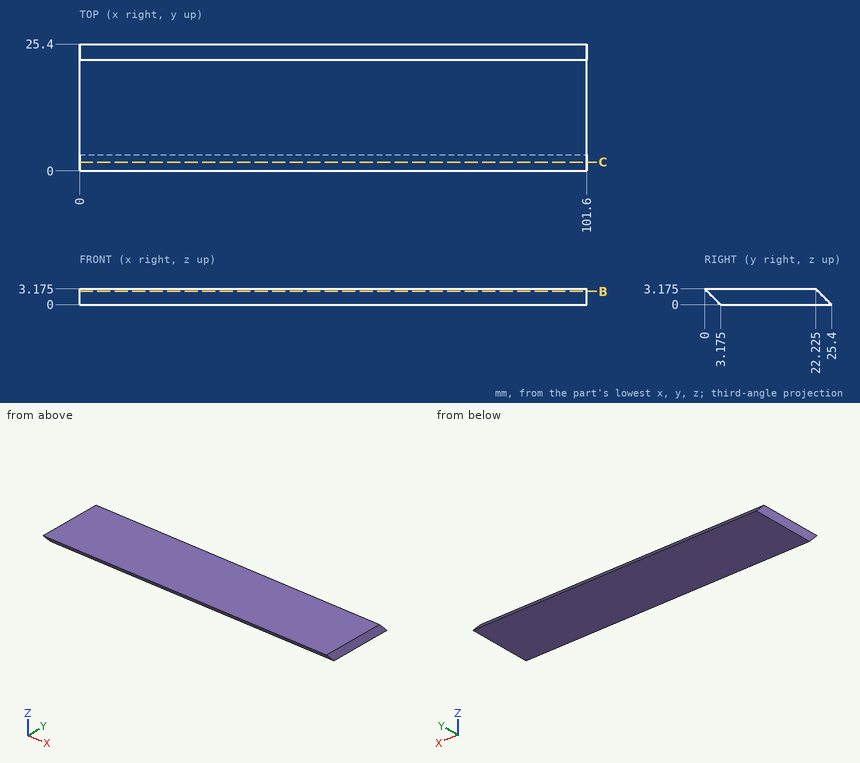
Could you check a few things on this drawing? It's one solid part, dimensions in mm from its lowest x, y, z. Give positions to 0.01 mm unless a question says otherwise; leave off trailing zeros. Order: outer loops, then holes, each group sorted by start corner. A loop starts at its lowest first (then second) coordinate and runs counter-clockwise, first axis right, second up. Notation, with made-up numbers: M 74.25,66 L 131.25,66 A30 cw 131.25,97 Z; hole C 62.5,89 d6. An arc over 180 degrees is marked long. Use one line per item in the form item = value. Start each with the question number.
Item 1: If we section it at B-B (z = 2.65): Write out the boundary of the cut face in (x, y) (3 decimals), then the cut area to 3 significant figures.
Item 2: If I drill on line 1 along Y through (x, z) = (50, 2.6) (3 decimals); line 2 along Z through (x, y) = (94, 22.75); line 3 along Z through (x, y) = (13, 1) (3 decimals), over which ranges is the centre line in solid material (lowest first)?
Item 3: If we section it at C-C (y = 1.75): Write out the boundary of the cut face in (x, z) (3 decimals), then the cut area to 3 significant figures.
Outcome:
q1.outline = M 0,0.525 L 101.6,0.525 L 101.6,22.75 L 0,22.75 Z
q1.area = 2,260 mm2
q2.line_1 = 0.575 to 22.8
q2.line_2 = 0 to 2.65
q2.line_3 = 2.175 to 3.175
q3.outline = M 0,1.425 L 101.6,1.425 L 101.6,3.175 L 0,3.175 Z
q3.area = 178 mm2
